from build123d import *

# Parameters (mm, degrees)
F1_DEPTH = 34.925
F2_D     = 3.556
F2_DEPTH = 34.926
F3_R     = 3.175
F4_DEPTH = 34.925


with BuildPart() as f1:
    # F0 (on Front) → F1 (new body, symmetric)
    with BuildSketch(Plane.XZ):
        Polygon((0, 0), (10.1648431926, 13.589), (-10.1648431926, 13.589), align=None)
        Polygon((-10.16, -13.5825253163), (10.16, -13.5825253163), (0, 0), align=None)
        with BuildLine():
            ThreePointArc((29.972, -40.068449683), (44.7411464985, -22.4060539587), (50.038, 0))
            ThreePointArc((50.038, 0), (44.7411464985, 22.4060539587), (29.972, 40.068449683))
            Line((29.972, 40.068449683), (10.1648431926, 13.589))
            Line((10.1648431926, 13.589), (0, 0))
            Line((0, 0), (10.16, -13.5825253163))
            Line((10.16, -13.5825253163), (29.972, -40.068449683))
        make_face()
        with BuildLine():
            Line((-10.1648431926, 13.589), (-29.972, 40.068449683))
            ThreePointArc((-29.972, 40.068449683), (-50.038, 0), (-29.972, -40.068449683))
            Line((-29.972, -40.068449683), (-10.16, -13.5825253163))
            Line((-10.16, -13.5825253163), (0, 0))
            Line((0, 0), (-10.1648431926, 13.589))
        make_face()
    extrude(amount=F1_DEPTH, both=True)

    # F2 (through all, one way)
    with BuildSketch(Plane.XZ):
        with Locations((0, 0)):
            Circle(F2_D / 2)
    extrude(amount=-F2_DEPTH, mode=Mode.SUBTRACT)

    # F3 (on Front) → F4 (cut, symmetric)
    with BuildSketch(Plane.XZ):
        Circle(F3_R)
    extrude(amount=F4_DEPTH, both=True, mode=Mode.SUBTRACT)


solid = f1.part
The model under review builds one solid part; all positions refer to its coordinate system, in mm. A direction names the side the tool comes from. Round coordinates to 2 decimals unless told otherwise and drop trailing zeros. Order: outer loops, then holes, each group sorted by start corner. A loop starts at its lowest first (then second) coordinate and runs counter-clockwise, first axis right, second up. Notation, with made-up numbers: (22.5, 54) -> (80.5, 54) arc R23 ccw to (80.5, 91) -> close; hole circle Ø2 at (81.25, 71). An arc over 180 degrees is marked (long way). Return JSON: item names as keys, results as strings.
1. Insertion check: P1, Ø10, axis at x = 39.5, y = 10.5, coming from the +Z side; P2, Ø8, axis at y = 6.5, z = -13, coming from the -X side; P3, Ø2, axis at x = -7.5, y = -4, coming from the -Z side. Each pin has a flat end and moves straight along its axis. Give the tip position at first contact, or say it passes through.
Answer block:
{"P1": "stops at z = 36.24", "P2": "stops at x = -49.22", "P3": "stops at z = -13.58"}
2. Take a section at C-C (z = 25). Write out the cut boundary in (x, y) (1 decimal).
Answer block:
{"outline": "(-43.3, -34.9) -> (-18.7, -34.9) -> (-18.7, 34.9) -> (-43.3, 34.9) -> close; (18.7, -34.9) -> (43.3, -34.9) -> (43.3, 34.9) -> (18.7, 34.9) -> close"}
3. For L1, parallel to Z at x = 0, y = 10 (3 decimals); L2, parallel to Z at x = 5.5, y = 10; L3, parallel to X at y = -19.5, z = -23, list the stretches that pass through material, from the lowest coordinate up. Write a range as [from, to].
Answer block:
{"L1": "z = [-13.583, -3.175], [3.175, 13.589]", "L2": "z = [-13.58, 13.59]", "L3": "x = [-44.44, -17.2], [17.2, 44.44]"}
4. For faces 1 (the face through (-1, -34.925, 9)), 2 (the face through (0, 0, 13.589)), 3 (the face through (-20.205, 0.489, -27.011)), list the 3-axis set-ups (+Z, -Z, +X, -X, +Y, -Y) from which the entire face can be reached by the end or side of a thin tool; tool diameter is ignored.
Answer block:
{"face 1": "+Z, -Z, +X, -X, -Y", "face 2": "+Z, +Y, -Y", "face 3": "-Z, +Y, -Y"}
5. Take a section at D-D (x = -33). Write out the cut boundary in (y, z) (3 decimals), then the cut area to 3 significant figures.
Answer block:
{"outline": "(-34.925, -37.614) -> (34.925, -37.614) -> (34.925, 37.614) -> (-34.925, 37.614) -> close", "area": "5,250 mm²"}
6. The part is to be moulded in two halves that separate along X. For faces 4 (the face through (-50.034, 0.489, 0.65)), 5 (the face through (20.207, -0.489, 27.014)), 6 (the face through (-1, 34.925, 9)), say which applies: +X half, -X half, draft (parallel to the pull), parting line (faces both ways), or undercut.
Answer block:
{"face 4": "-X half", "face 5": "undercut", "face 6": "draft"}
7. Take a section at B-B (y = 6). Write out the cut boundary in (x, z) (3 decimals).
Answer block:
{"outline": "(-29.972, -40.068) -> (-10.16, -13.583) -> (10.16, -13.583) -> (29.972, -40.068) arc R50.038 ccw to (29.972, 40.068) -> (10.165, 13.589) -> (-10.165, 13.589) -> (-29.972, 40.068) arc R50.038 ccw to start; hole circle Ø6.35 at (0, 0)"}
8. Take a section at A-A (x = 0). Write out the cut boundary in (y, z) (3 decimals), then the cut area to 3 significant figures.
Answer block:
{"outline": "(-34.925, -13.583) -> (34.925, -13.583) -> (34.925, -3.175) -> (-34.925, -3.175) -> close; (-34.925, 3.175) -> (34.925, 3.175) -> (34.925, 13.589) -> (-34.925, 13.589) -> close", "area": "1,450 mm²"}
